from build123d import *

# Parameters (mm, degrees)
BOSS_EXTRUDE1_DEPTH  = 25.4
SKETCH7_W            = 35.937578614
SKETCH7_H            = 7.62
BOSS_EXTRUDE3_DEPTH  = 40.95
SKETCH8_W            = 6.35
SKETCH8_H            = 35.937578614
BOSS_EXTRUDE4_DEPTH  = 35
SKETCH9_W            = 7.62
SKETCH9_H            = 35.937578614
BOSS_EXTRUDE5_DEPTH  = 25.4
BOSS_EXTRUDE6_REACH  = 135.462
SKETCH10_W           = 35.937578614
SKETCH10_H           = 5.08
CUT_EXTRUDE1_REACH   = 172.448
SKETCH11_W           = 16.51
SKETCH11_H           = 7.62
BOSS_EXTRUDE7_DEPTH  = 2.162419
SKETCH14_W           = 50.8
SKETCH14_H           = 25.4
BOSS_EXTRUDE9_DEPTH  = 2.54
M6_CLEARANCE_HOLE2_D = 7
CUT_EXTRUDE2_REACH   = 171.327
SKETCH18_R           = 1.651
SKETCH19_W           = 7.62
SKETCH19_H           = 16.51
CUT_EXTRUDE4_DEPTH   = 1.27


with BuildPart() as part:
    # Sketch1 → Boss-Extrude1 (new body)
    with BuildSketch(Plane(origin=(0, 0, 0), x_dir=(1, 0, 0), z_dir=(0, 1, 0))):
        Polygon((6.35, 4.219850082), (-24.6, 54.359549401), (-24.6, 90.297128015), (-32.22, 90.297128015), (-32.22, 52.197128015), (0, 0), (6.35, 0), align=None)
    extrude(amount=BOSS_EXTRUDE1_DEPTH)

    # Sketch7 → Boss-Extrude3 (add)
    with BuildSketch(Plane(origin=(-24.6, 0, 0), x_dir=(0, 0, -1), z_dir=(1, 0, 0))):
        with Locations((72.328338708, 3.81)):
            Rectangle(SKETCH7_W, SKETCH7_H)
    extrude(amount=BOSS_EXTRUDE3_DEPTH)

    # Sketch8 → Boss-Extrude4 (add)
    with BuildSketch(Plane.XZ):
        with Locations((13.175, -72.328338708)):
            Rectangle(SKETCH8_W, SKETCH8_H)
    extrude(amount=BOSS_EXTRUDE4_DEPTH)


with BuildPart() as body_2:
    # Mirror6: mirrored copy
    add(part.part.mirror(Plane.ZY.offset(50)))


with BuildPart() as part_1:
    add(part.part)

    add(body_2.part)  # Boss-Extrude5 merges body 2
    # Sketch9 → Boss-Extrude5 (add)
    with BuildSketch(Plane(origin=(0, 25.4, 0), x_dir=(1, 0, 0), z_dir=(0, 1, 0))):
        with Locations((-71.59, 72.328338708)):
            Rectangle(SKETCH9_W, SKETCH9_H)
        with Locations((-28.41, 72.328338708)):
            Rectangle(SKETCH9_W, SKETCH9_H)
    extrude(amount=BOSS_EXTRUDE5_DEPTH)

    # Sketch10 → Boss-Extrude6 (add, up to next)
    with BuildSketch(Plane(origin=(-67.78, 0, 0), x_dir=(0, 0, -1), z_dir=(1, 0, 0)), mode=Mode.PRIVATE) as boss_extrude6_sk1:
        with Locations((72.328338708, 48.26)):
            Rectangle(SKETCH10_W, SKETCH10_H)
    boss_extrude6_tool1 = extrude(boss_extrude6_sk1.sketch, amount=BOSS_EXTRUDE6_REACH, mode=Mode.PRIVATE) - part_1.part
    add(boss_extrude6_tool1.solids().sort_by_distance((-67.78, 48.26, -72.328339))[0])

    # Sketch11 → Cut-Extrude1 (cut, up to next)
    with BuildSketch(Plane(origin=(0, 50.8, 0), x_dir=(1, 0, 0), z_dir=(0, 1, 0)), mode=Mode.PRIVATE) as cut_extrude1_sk1:
        with Locations((-50, 58.169549401)):
            Rectangle(SKETCH11_W, SKETCH11_H)
    cut_extrude1_tool1 = extrude(cut_extrude1_sk1.sketch, amount=-CUT_EXTRUDE1_REACH, mode=Mode.PRIVATE) & part_1.part
    # Sketch11 → Cut-Extrude1 (cut, up to next)
    with BuildSketch(Plane(origin=(0, 50.8, 0), x_dir=(1, 0, 0), z_dir=(0, 1, 0)), mode=Mode.PRIVATE) as cut_extrude1_sk2:
        with Locations((-50, 86.487128015)):
            Rectangle(SKETCH11_W, SKETCH11_H)
    cut_extrude1_tool2 = extrude(cut_extrude1_sk2.sketch, amount=-CUT_EXTRUDE1_REACH, mode=Mode.PRIVATE) & part_1.part
    add(cut_extrude1_tool1.solids().sort_by_distance((-50, 50.8, -58.169549))[0], mode=Mode.SUBTRACT)
    add(cut_extrude1_tool2.solids().sort_by_distance((-50, 50.8, -86.487128))[0], mode=Mode.SUBTRACT)

    # Sketch12 → Boss-Extrude7 (add)
    with BuildSketch(Plane.XY.offset(-54.359549401)):
        Polygon((-75.4, 50.8), (-24.6, 50.8), (-24.6, 25.4), (-32.22, 25.4), (-32.22, 45.72), (-67.78, 45.72), (-67.78, 25.4), (-75.4, 25.4), align=None)
    extrude(amount=BOSS_EXTRUDE7_DEPTH)

    # Sketch14 → Boss-Extrude9 (add)
    with BuildSketch(Plane(origin=(0, 0, -90.297128015), x_dir=(-1, 0, 0), z_dir=(0, 0, -1))):
        with Locations((50, 38.1)):
            Rectangle(SKETCH14_W, SKETCH14_H)
    extrude(amount=BOSS_EXTRUDE9_DEPTH)

    # M6 Clearance Hole2 (through all)
    with Locations(Plane(origin=(16.35, 0, 0), x_dir=(0, 0, -1), z_dir=(1, 0, 0))):
        with Locations((72.633968015, -17.78)):
            Hole(M6_CLEARANCE_HOLE2_D / 2)

    # Sketch18 → Cut-Extrude2 (cut, up to next)
    with BuildSketch(Plane(origin=(0, 45.72, 0), x_dir=(-1, 0, 0), z_dir=(0, -1, 0)), mode=Mode.PRIVATE) as cut_extrude2_sk1:
        with Locations(Location((37.080244901, 58.064528015, 0), (0, 0, 90))):
            Circle(SKETCH18_R)
    cut_extrude2_tool1 = extrude(cut_extrude2_sk1.sketch, amount=-CUT_EXTRUDE2_REACH, mode=Mode.PRIVATE) & part_1.part
    # Sketch18 → Cut-Extrude2 (cut, up to next)
    with BuildSketch(Plane(origin=(0, 45.72, 0), x_dir=(-1, 0, 0), z_dir=(0, -1, 0)), mode=Mode.PRIVATE) as cut_extrude2_sk2:
        with Locations(Location((63.445444901, 58.064528015, 0), (0, 0, 90))):
            Circle(SKETCH18_R)
    cut_extrude2_tool2 = extrude(cut_extrude2_sk2.sketch, amount=-CUT_EXTRUDE2_REACH, mode=Mode.PRIVATE) & part_1.part
    # Sketch18 → Cut-Extrude2 (cut, up to next)
    with BuildSketch(Plane(origin=(0, 45.72, 0), x_dir=(-1, 0, 0), z_dir=(0, -1, 0)), mode=Mode.PRIVATE) as cut_extrude2_sk3:
        with Locations(Location((63.445444901, 84.429728015, 0), (0, 0, 90))):
            Circle(SKETCH18_R)
    cut_extrude2_tool3 = extrude(cut_extrude2_sk3.sketch, amount=-CUT_EXTRUDE2_REACH, mode=Mode.PRIVATE) & part_1.part
    # Sketch18 → Cut-Extrude2 (cut, up to next)
    with BuildSketch(Plane(origin=(0, 45.72, 0), x_dir=(-1, 0, 0), z_dir=(0, -1, 0)), mode=Mode.PRIVATE) as cut_extrude2_sk4:
        with Locations(Location((37.080244901, 84.429728015, 0), (0, 0, 90))):
            Circle(SKETCH18_R)
    cut_extrude2_tool4 = extrude(cut_extrude2_sk4.sketch, amount=-CUT_EXTRUDE2_REACH, mode=Mode.PRIVATE) & part_1.part
    add(cut_extrude2_tool1.solids().sort_by_distance((-37.080245, 45.72, -58.064528))[0], mode=Mode.SUBTRACT)
    add(cut_extrude2_tool2.solids().sort_by_distance((-63.445445, 45.72, -58.064528))[0], mode=Mode.SUBTRACT)
    add(cut_extrude2_tool3.solids().sort_by_distance((-63.445445, 45.72, -84.429728))[0], mode=Mode.SUBTRACT)
    add(cut_extrude2_tool4.solids().sort_by_distance((-37.080245, 45.72, -84.429728))[0], mode=Mode.SUBTRACT)

    # Sketch19 → Cut-Extrude4 (cut)
    with BuildSketch(Plane.XZ.offset(-45.72)):
        with Locations((-38.316, -72.327898015)):
            Rectangle(SKETCH19_W, SKETCH19_H)
        with Locations((-61.684, -72.327898015)):
            Rectangle(SKETCH19_W, SKETCH19_H)
    extrude(amount=-CUT_EXTRUDE4_DEPTH, mode=Mode.SUBTRACT)


solid = part_1.part
Source: CAD feature listing. Evaluate the final solid. Frame: model axes, mm. A direction names the side the tool comes from. Give positions to 0.01 mm unless a question says otherwise; leave off trailing zeros. Write each loop counter-clockwise with the first axis right and the second up, starting at its lowest first coordinate (ties: lowest second). Pieces come first, ordered by that corner, then holes. Notation, with made-up numbers: M 74.5,8 L 87.5,8 A29 ccw 87.5,31 Z; hole C -26.75,45.5 d4. An arc over 180 degrees is marked long. Return JSON: item names as keys, results as strings. Group by question number.
1) First-contact query: pin 1 Ø19.5 at (x, z) = (-85.5, -18.5) entering from +Y; pin 2 Ø6 at (x, y) = (-91, 21.5) entering from -Z; pin 3 Ø21 at (x, z) = (-79.5, -27) entering from -Y. Flat tips, straight axial feed; report the tip coordinate or a pass-through.
2) Draft query along X for faces 1 (the face through (-75.4, 29, -72)), 2 (the face through (-50, 48, -54.36)), 3 (the face through (-67.78, 23, -72)), 4 (the face through (3, 13, 0)). Return one class per face: released by +X, released by -X, zero draft, split by the parting line, or undercut.
3) Cut plane B-B, the plane z = -29. Output: boundary loops of the cut face in (x, y).
4) Set-up query: faces 5 (the face through (-110, -13, -73)), 6 (the face through (-50, 47, -52.197)), 7 (the face through (-8.91, 12.52, -28.94)), 8 (the face through (-96, 2, -90.297)). Return all of +Z, -Z, +X, -X, +Y, -Y with unobstructed straight access to the full face (end or side cutting, diameter ignored); none if empty.
5) Cut plane A-A, the plane y = -24. Output: boundary loops of the cut face in (x, z), then the cut area to 3 significant figures.
6) Cut plane D-D, the plane z = -73.5. Give the number of separate pieces and of enclosed holes in the cut face, then the cut area to 3 significant figures.
7) Cut plane C-C, the plane x = -44.5. Output: boundary loops of the cut face in (y, z).
8) Ray query, L1, parallel to X at y = -25, z = -68; L2, parallel to Y at x = -88.5, z = -65.5; L3, parallel to X at y = 1, z = -62.5. Return the intervals inside material, ascending.
Data:
{
 "1": {"pin 1": "stops at y = 25.4", "pin 2": "stops at z = -33.95", "pin 3": "stops at y = 0"},
 "2": {"face 1": "released by -X", "face 2": "undercut", "face 3": "undercut", "face 4": "zero draft"},
 "3": {"outline": "M -91.05,0 L -82.1,0 L -82.1,25.4 L -91.05,25.4 Z; M -17.9,0 L -8.95,0 L -8.95,25.4 L -17.9,25.4 Z"},
 "4": {"face 5": "+Z, -Z, -Y", "face 6": "+Z, +X, -X, +Y", "face 7": "+X, +Y, -Y", "face 8": "-Z, +X, -X, -Y"},
 "5": {"outline": "M -116.35,-90.3 L -110,-90.3 L -110,-54.36 L -116.35,-54.36 Z; M 10,-90.3 L 16.35,-90.3 L 16.35,-54.36 L 10,-54.36 Z", "area": "456 mm²"},
 "6": {"separate pieces": "3", "enclosed holes": "0", "area": "1,920 mm²"},
 "7": {"outline": "M 25.4,-92.84 L 50.8,-92.84 L 50.8,-90.3 L 25.4,-90.3 Z; M 45.72,-82.68 L 50.8,-82.68 L 50.8,-61.98 L 45.72,-61.98 Z; M 45.72,-54.36 L 50.8,-54.36 L 50.8,-52.2 L 45.72,-52.2 Z"},
 "8": {"L1": "x = -116.35 to -110, 10 to 16.35", "L2": "y = 0 to 7.62", "L3": "x = -116.35 to -67.78, -32.22 to 16.35"}
}
